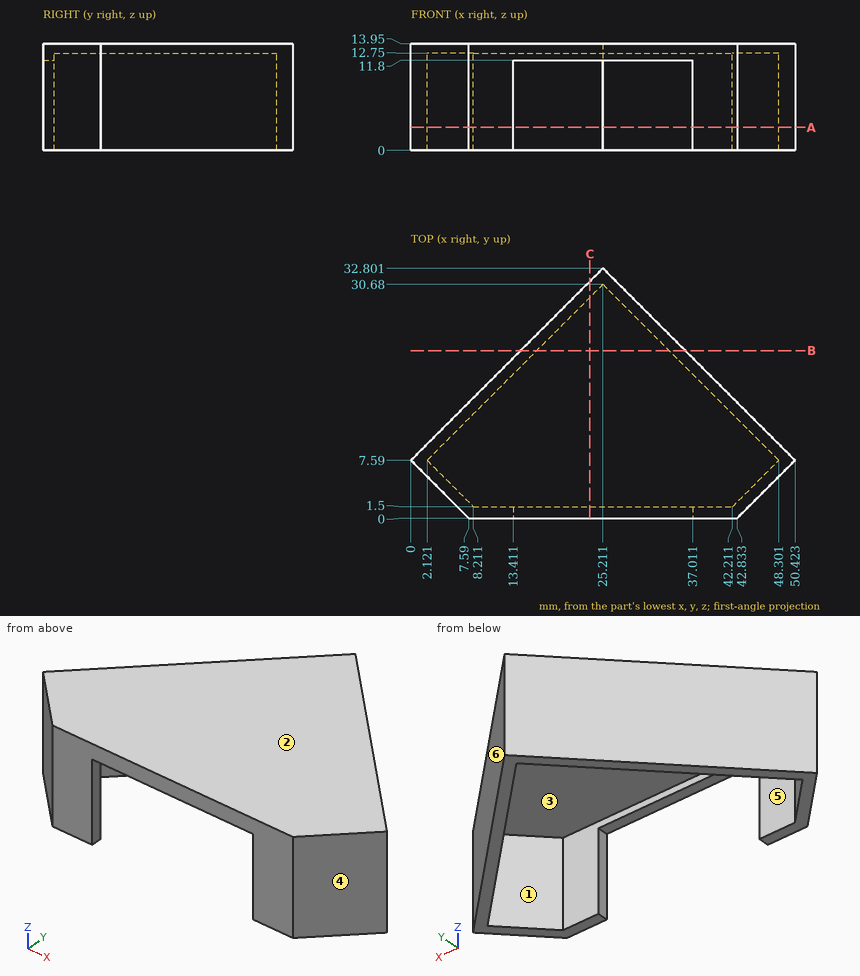
Can you work these out from the drawing? Everything is in mm from the part's minimum corner. A direction names the side the tool comes from. Round coordinates to 2 decimals unless told otherwise and drop trailing zeros. Loops run counter-clockwise (first coordinate to the right, second up) from the corner with the lowest first, then second, coordinate; pieces in that order, holes last. Notation, with made-up numbers: (58.25, 66) - (63.25, 66) arc R24 ccw to (63.25, 85) - close; hole circle Ø9 at (83.5, 11.5). An arc over 180 degrees is marked (long way). Answer in a Markdown table with one row per item. Add a question column.
(1) For the marked faces 5 and 6, which set-ups out of +Z, -Z, +X, -X, +Y, -Y let a thin tool reach every point of the face, with its end or its side?
(2) I need wall thicknesses on line 1 along X through (y, z) = (17.5, 9.25) (1 decimal); line 2 along Y through (x, z) = (38.5, 4.5) (1 decimal); line 3 along X through (y, z) = (22.5, 5.25) (1 decimal). Which ranges of each line are inside material? Lowest first, please.
(3) If we section it at A-A (z = 3): Please give me the cut outline in (x, y).
(4) If we section it at C-C (x = 23.5): Please give me the cut outline in (y, z).
(5) If we mould it in two halves opening along Y, with no side actions, what happens to the marked faces 1, 2, 3 and 4? For each: pulls with the +Y half, pulls with the -Y half, needs draft (parallel to the pull), parting line crosses it, or undercut.
(6) If we section it at B-B (y = 22): Please give me the cut outline in (x, z).
(7) I'm going to push flat-ended pins straight in: pin 1 (1.5 mm diameter, centred on x = 22, z = 6.5, fed in from +Y); pin 2 (8 mm diameter, centred on y = 22, z = 11, fed in from -X); pin 3 (1.5 mm diameter, centred on y = 14.5, z = 6.5, fed in from -X); pin 4 (5 mm diameter, centred on x = 27, z = 6, fed in from +Y). Where does each tip first touch, or does it pass through?
Model answer:
| question | item | result |
|---|---|---|
| 1 | face 5 | -Z |
| 1 | face 6 | +Z, -Z, +X, +Y |
| 2 | line 1 | x = 9.9 to 12, 38.4 to 40.5 |
| 2 | line 2 | y = 0 to 1.5, 17.4 to 19.5 |
| 2 | line 3 | x = 14.9 to 17, 33.4 to 35.5 |
| 3 | outline | (0, 7.59) - (7.59, 0) - (13.41, 0) - (13.41, 1.5) - (8.21, 1.5) - (2.12, 7.59) - (25.21, 30.68) - (48.3, 7.59) - (42.21, 1.5) - (37.01, 1.5) - (37.01, 0) - (42.83, 0) - (50.42, 7.59) - (25.21, 32.8) - close |
| 4 | outline | (0, 11.8) - (1.5, 11.8) - (1.5, 12.75) - (28.97, 12.75) - (28.97, 0) - (31.09, 0) - (31.09, 13.95) - (0, 13.95) - close |
| 5 | face 1 | undercut |
| 5 | face 2 | needs draft |
| 5 | face 3 | undercut |
| 5 | face 4 | pulls with the -Y half |
| 6 | outline | (14.41, 0) - (16.53, 0) - (16.53, 12.75) - (33.89, 12.75) - (33.89, 0) - (36.01, 0) - (36.01, 13.95) - (14.41, 13.95) - close |
| 7 | pin 1 | stops at y = 30.34 |
| 7 | pin 2 | stops at x = 10.41 |
| 7 | pin 3 | stops at x = 6.16 |
| 7 | pin 4 | stops at y = 32.8 |
